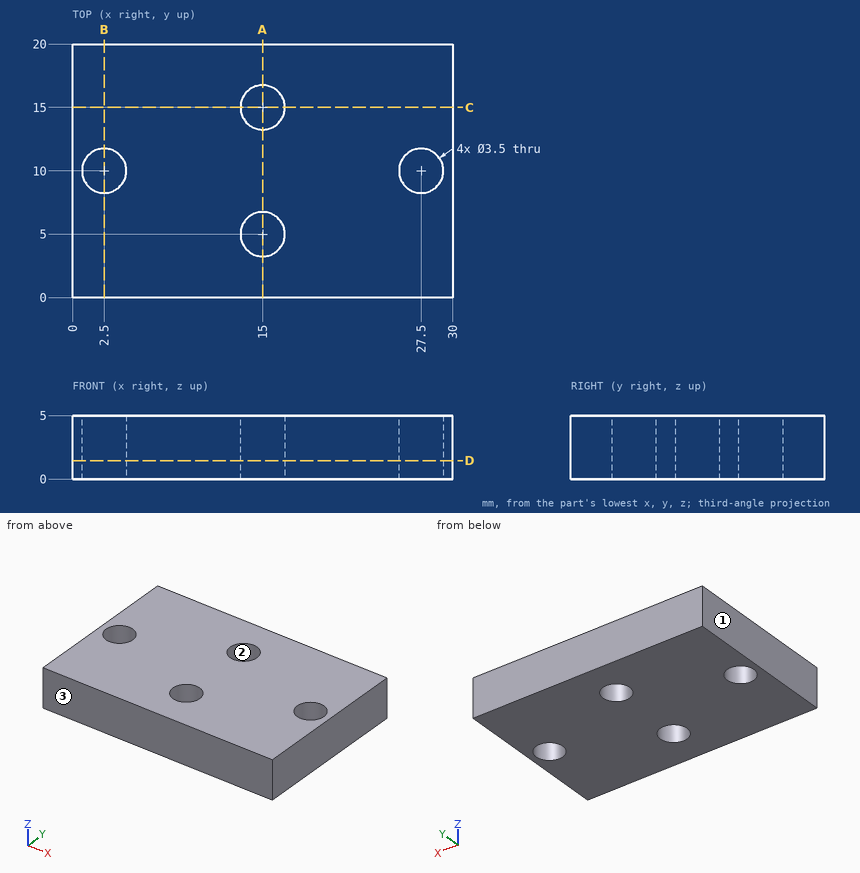
The drawing under review shows one solid part. Ordinate dimensions are in mm from its lowest x, y, z. Coordinates: 2 decimals unless noted, no trailing zeros. Order: outer loops, then holes, each group sorted by start corner. A loop starts at its lowest first (then second) coordinate and runs counter-clockwise, first axis right, second up. Notation, with made-up numbers: M -12,-10 L 42,-10 A22 cw 42,23 Z; hole C -29.75,48 d1. An arc over 180 degrees is marked long. Use a Markdown table: item, result.
(1) Draft analysis for pull direction Y (two halves, no side actions). For the marked faces 1, 2 and 3, state which applies: released by +Y, released by -Y, zero draft, split by the parting line, or undercut.
Worked answers:
| item | result |
|---|---|
| face 1 | zero draft |
| face 2 | undercut |
| face 3 | released by -Y |
(2) Add section A-A (x = 15). Give the boundary of the cut face in (y, z).
Worked answers:
| item | result |
|---|---|
| outline | M 0,0 L 3.25,0 L 3.25,5 L 0,5 Z; M 6.75,0 L 13.25,0 L 13.25,5 L 6.75,5 Z; M 16.75,0 L 20,0 L 20,5 L 16.75,5 Z |
(3) Add section D-D (z = 1.45). Give the boundary of the cut face in (x, y), then the cut area to 3 significant figures.
Worked answers:
| item | result |
|---|---|
| outline | M 0,0 L 30,0 L 30,20 L 0,20 Z; hole C 2.5,10 d3.5; hole C 15,5 d3.5; hole C 15,15 d3.5; hole C 27.5,10 d3.5 |
| area | 562 mm2 |
(4) Wall thickness on probe 1 along Y at (x, z) = (15, 3.5); probe 2 along Y at (x, z) = (2.5, 2.2); probe 3 along Y at (x, z) = (13.75, 1.75): over which ranges is each line inside the solid? List them lowest first.
Worked answers:
| item | result |
|---|---|
| probe 1 | y = 0 to 3.25, 6.75 to 13.25, 16.75 to 20 |
| probe 2 | y = 0 to 8.25, 11.75 to 20 |
| probe 3 | y = 0 to 3.78, 6.22 to 13.78, 16.22 to 20 |
(5) Add section C-C (y = 15). Give the boundary of the cut face in (x, z), then the cut area to 4 significant figures.
Worked answers:
| item | result |
|---|---|
| outline | M 0,0 L 13.25,0 L 13.25,5 L 0,5 Z; M 16.75,0 L 30,0 L 30,5 L 16.75,5 Z |
| area | 132.5 mm2 |
(6) Add section B-B (x = 2.5). Give the boundary of the cut face in (y, z), then the cut area to 3 significant figures.
Worked answers:
| item | result |
|---|---|
| outline | M 0,0 L 8.25,0 L 8.25,5 L 0,5 Z; M 11.75,0 L 20,0 L 20,5 L 11.75,5 Z |
| area | 82.5 mm2 |
